```python
from build123d import *

# Parameters (mm, degrees)
ESQUISSE1_W                     = 20
ESQUISSE1_H                     = 20
BOSS_EXTRU_1_DEPTH              = 10
ESQUISSE2_W                     = 237.218260139
ESQUISSE2_H                     = 128.428413156
ENL_V_MAT_EXTRU_6_DEPTH         = 10
ENL_V_MAT_EXTRU_7_DEPTH         = 10
BOSS_EXTRU_4_START              = -2
BOSS_EXTRU_4_DEPTH              = 9
ESQUISSE10_W                    = 2
ESQUISSE10_H                    = 4
BOSS_EXTRU_5_DEPTH              = 224.980719072
ESQUISSE11_W                    = 2.5
ESQUISSE11_H                    = 5
BOSS_EXTRU_6_DEPTH              = 4
SYM_TRIE1_START                 = 8
SYM_TRIE1_OUTLINE_W             = 4
SYM_TRIE1_OUTLINE_H             = 4
SYM_TRIE1_DEPTH                 = 9
BOSS_EXTRU_9_REACH              = 128.238
BOSS_EXTRU_9_DIRECTION_2_REACH  = 128.238
BOSS_EXTRU_10_REACH             = 128.238
BOSS_EXTRU_10_DIRECTION_2_REACH = 128.238
ESQUISSE14_W                    = 8
ESQUISSE14_H                    = 8
BOSS_EXTRU_11_DEPTH             = 25


# Read off the part's stored shape, not the designer's step: Sym_trie1
with BuildPart() as part:
    # Esquisse1 → Boss.-Extru.1 (new body)
    with BuildSketch(Plane.XY):
        Polygon((-116.245179768, 65.5), (-116.245179768, 40.5), (-116.189357624, -40.5), (-116.189357624, -65.5), (108.67971716, -65.5), (108.67971716, -40.5), (108.735539304, 40.5), (108.735539304, 65.5), align=None)
        Polygon((83.754820232, 40.5), (106.172004788, 40.5), (106.172004788, -40.5), (83.67971716, -40.5), (83.67971716, -63), (-91.189357624, -63), (-91.189357624, -40.5), (-113.681645253, -40.5), (-113.681645253, 40.5), (-91.264460696, 40.5), (-91.264460696, 63), (83.754820232, 63), align=None, mode=Mode.SUBTRACT)
        Polygon((-113.66622051, -63.007706414), (-113.681645253, -43.007712371), (-93.681645253, -43.023131157), (-93.697069995, -62.992287629), align=None, mode=Mode.SUBTRACT)
        Polygon((106.172004788, -43.007712371), (106.156580046, -63.007706414), (86.187429531, -62.992287629), (86.172004788, -43.023131157), align=None, mode=Mode.SUBTRACT)
        with Locations((-103.754820232, 53)):
            Rectangle(ESQUISSE1_W, ESQUISSE1_H, mode=Mode.SUBTRACT)
        with Locations((96.245179768, 53)):
            Rectangle(ESQUISSE1_W, ESQUISSE1_H, mode=Mode.SUBTRACT)
    extrude(amount=BOSS_EXTRU_1_DEPTH)

    # Esquisse2 → Enl_v. mat.-Extru.6 (cut)
    with BuildSketch(Plane(origin=(0, 0, 0), x_dir=(-1, 0, 0), z_dir=(0, 0, -1))):
        with Locations((9.873590765, -23.714206578)):
            Rectangle(ESQUISSE2_W, ESQUISSE2_H)
    extrude(amount=-ENL_V_MAT_EXTRU_6_DEPTH, mode=Mode.SUBTRACT)

    # Esquisse4 → Enl_v. mat.-Extru.7 (cut)
    with BuildSketch(Plane(origin=(0, 0, 0), x_dir=(-1, 0, 0), z_dir=(0, 0, -1))):
        Polygon((-83.754820232, 63), (-83.754820232, 68.626436571), (91.264460696, 65.5), (91.264460696, 63), align=None)
    extrude(amount=-ENL_V_MAT_EXTRU_7_DEPTH, mode=Mode.SUBTRACT)


with BuildPart() as enl_v_mat_extru_7_piece_1:
    # of the separate pieces the step leaves, piece 1, a body of its own (enl_v_mat_extru_7_pieces)
    add(part.part.solids().sort_by_distance((-116.245179768, 65.5, 0))[0])

    # Esquisse9 → Boss.-Extru.4 (add)
    with BuildSketch(Plane.XY.offset(10).offset(BOSS_EXTRU_4_START)):
        Polygon((-116.245179768, 53), (-116.245179768, 55), (-120.245179768, 55), (-120.245179768, 51), (-116.245179768, 51), align=None)
    extrude(amount=BOSS_EXTRU_4_DEPTH)

    # Esquisse10 → Boss.-Extru.5 (add)
    with BuildSketch(Plane(origin=(-116.245179768, 0, 0), x_dir=(0, 0, -1), z_dir=(1, 0, 0))):
        with Locations((-16, 53)):
            Rectangle(ESQUISSE10_W, ESQUISSE10_H)
    extrude(amount=BOSS_EXTRU_5_DEPTH)

    # Esquisse11 → Boss.-Extru.6 (add)
    with BuildSketch(Plane.XZ.offset(-51)):
        with Locations((-114.995179768, 12.5)):
            Rectangle(ESQUISSE11_W, ESQUISSE11_H)
    extrude(amount=-BOSS_EXTRU_6_DEPTH)

    # Sym_trie1 outline → Sym_trie1 (add)
    with BuildSketch(Plane.XY.offset(SYM_TRIE1_START)):
        with Locations((-122.245179768, 53)):
            Rectangle(SYM_TRIE1_OUTLINE_W, SYM_TRIE1_OUTLINE_H)
    extrude(amount=SYM_TRIE1_DEPTH)


with BuildPart() as enl_v_mat_extru_7_piece_2:
    # of the separate pieces the step leaves, piece 2, a body of its own (enl_v_mat_extru_7_pieces)
    add(part.part.solids().sort_by_distance((108.735539304, 65.5, 0))[0])

    # Boss.-Extru.9: up to this face of the body (flat: up to its plane)
    boss_extru_9_end = Plane(enl_v_mat_extru_7_piece_2.part.faces().sort_by_distance((96.245179768, 65.5, 5))[0])
    # Esquisse12 → Boss.-Extru.9 (add, up to the picked face)
    with BuildSketch(Plane(origin=(0, 55, 0), x_dir=(1, 0, 0), z_dir=(0, 1, 0)), mode=Mode.PRIVATE) as boss_extru_9_sk1:
        Polygon((108.735539304, -10), (108.735539304, -8), (116.735539304, -8), (116.735539304, -17), (108.735539304, -17), (108.735539304, -15), (106.245539304, -15), (106.245539304, -10), align=None)
    boss_extru_9_tool1 = split(extrude(boss_extru_9_sk1.sketch, amount=BOSS_EXTRU_9_REACH, mode=Mode.PRIVATE), bisect_by=boss_extru_9_end, keep=Keep.BOTH, mode=Mode.PRIVATE)

    add(enl_v_mat_extru_7_piece_1.part)  # Boss.-Extru.9 merges Enl_v. mat.-Extru.7 piece 1
    add(boss_extru_9_tool1.solids().sort_by(Axis((111.962298, 55, 12.5), (0, 1, 0)))[0])

    # Boss.-Extru.9 direction 2: up to this face of the body (flat: up to its plane)
    boss_extru_9_direction_2_end = Plane(enl_v_mat_extru_7_piece_2.part.faces().sort_by_distance((96.245179768, 40.5, 5))[0])
    # Esquisse12 → Boss.-Extru.9 direction 2 (add, up to the picked face)
    with BuildSketch(Plane(origin=(0, 55, 0), x_dir=(1, 0, 0), z_dir=(0, 1, 0)), mode=Mode.PRIVATE) as boss_extru_9_direction_2_sk1:
        Polygon((108.735539304, -10), (108.735539304, -8), (116.735539304, -8), (116.735539304, -17), (108.735539304, -17), (108.735539304, -15), (106.245539304, -15), (106.245539304, -10), align=None)
    boss_extru_9_direction_2_tool1 = split(extrude(boss_extru_9_direction_2_sk1.sketch, amount=-BOSS_EXTRU_9_DIRECTION_2_REACH, mode=Mode.PRIVATE), bisect_by=boss_extru_9_direction_2_end, keep=Keep.BOTH, mode=Mode.PRIVATE)
    add(boss_extru_9_direction_2_tool1.solids().sort_by(Axis((111.962298, 55, 12.5), (0, -1, 0)))[0])

    # Boss.-Extru.10: up to this face of the body (flat: up to its plane)
    boss_extru_10_end = Plane(enl_v_mat_extru_7_piece_2.part.faces().sort_by_distance((100.216105898, 65.5, 6.894873222))[0])
    # Esquisse13 → Boss.-Extru.10 (add, up to the picked face)
    with BuildSketch(Plane(origin=(0, 55, 0), x_dir=(1, 0, 0), z_dir=(0, 1, 0)), mode=Mode.PRIVATE) as boss_extru_10_sk1:
        Polygon((-124.245179768, -17), (108.735539304, -17), (108.735539304, -15), (-113.745179768, -15), (-113.745179768, -10), (-116.245179768, -10), (-116.245179768, -8), (-124.245179768, -8), align=None)
    boss_extru_10_tool1 = split(extrude(boss_extru_10_sk1.sketch, amount=BOSS_EXTRU_10_REACH, mode=Mode.PRIVATE), bisect_by=boss_extru_10_end, keep=Keep.BOTH, mode=Mode.PRIVATE)
    add(boss_extru_10_tool1.solids().sort_by(Axis((-22.049518, 55, 15.446639), (0, 1, 0)))[0])

    # Boss.-Extru.10 direction 2: up to this face of the body (flat: up to its plane)
    boss_extru_10_direction_2_end = Plane(enl_v_mat_extru_7_piece_2.part.faces().sort_by_distance((-103.754820232, 40.5, 5))[0])
    # Esquisse13 → Boss.-Extru.10 direction 2 (add, up to the picked face)
    with BuildSketch(Plane(origin=(0, 55, 0), x_dir=(1, 0, 0), z_dir=(0, 1, 0)), mode=Mode.PRIVATE) as boss_extru_10_direction_2_sk1:
        Polygon((-124.245179768, -17), (108.735539304, -17), (108.735539304, -15), (-113.745179768, -15), (-113.745179768, -10), (-116.245179768, -10), (-116.245179768, -8), (-124.245179768, -8), align=None)
    boss_extru_10_direction_2_tool1 = split(extrude(boss_extru_10_direction_2_sk1.sketch, amount=-BOSS_EXTRU_10_DIRECTION_2_REACH, mode=Mode.PRIVATE), bisect_by=boss_extru_10_direction_2_end, keep=Keep.BOTH, mode=Mode.PRIVATE)
    add(boss_extru_10_direction_2_tool1.solids().sort_by(Axis((-22.049518, 55, 15.446639), (0, -1, 0)))[0])

    # Esquisse14 → Boss.-Extru.11 (add)
    with BuildSketch(Plane(origin=(0, 65.5, 0), x_dir=(1, 0, 0), z_dir=(0, 1, 0))):
        with Locations((112.735539304, -4)):
            Rectangle(ESQUISSE14_W, ESQUISSE14_H)
        with Locations((-120.245179768, -4)):
            Rectangle(ESQUISSE14_W, ESQUISSE14_H)
    extrude(amount=-BOSS_EXTRU_11_DEPTH)


solid = enl_v_mat_extru_7_piece_2.part
```
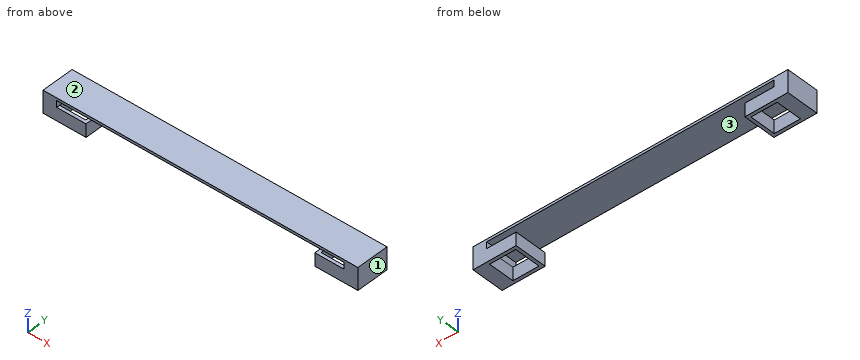
Geometry: final body of the model. Coordinates: model frame, mm. Face numbers are marked on the shaded views. Give positions to 0.01 mm unless a question says otherwise; leave off trailing zeros. Write each loop counter-clockwise with the first axis right and the second up, starting at its lowest first coordinate (ties: lowest second). Pieces come first, ordered by that corner, then holes.
1. Draft query along X for the marked faces 1, 2 and 3. Return one class per face: released by +X, released by -X, zero draft, split by the parting line, or undercut.
2. Section query B-B, the plane z = 12.5. Return loops of the section in (x, y).
3. Pin query (flat end, axial travel): P1, Ø6, axis at x = -85.5, z = 7, coming from the -Y side; P2, Ø12.5, axis at x = -58, y = 53, coming from the -Z side. Return the tip coordinate at first contact, or that it passes through.
4. Line query: probe 1 along X at (y, z) = (48.75, 5); probe 2 along X at (y, z) = (43.75, 12); probe 3 along Z at (x, y) = (-93, 45.25). Output: solid intervals per line, ascending.
5. Section query A-A, the plane x = -100. Return loops of the section in (y, z), then the cut area to 4 significant figures.
6. Section query C-C, the plane y = 49. Count the separate pieces of the cut face and the enclosed holes in it, then the cut area to 3 significant figures.
7. Section query D-D, the plane x = -14. Return loops of the section in (y, z).
Computed:
1. face 1: released by +X
1. face 2: zero draft
1. face 3: undercut
2. outline: (-124.25, 40.5) - (-113.75, 40.5) - (-113.75, 65.5) - (-124.25, 65.5) - close; (106.25, 40.5) - (116.74, 40.5) - (116.74, 65.5) - (106.25, 65.5) - close
3. P1: passes through
3. P2: stops at z = 15
4. probe 1: x = -124.25 to -113.75, -93.75 to -91.26, 83.75 to 86.25, 106.25 to 116.74
4. probe 2: x = -124.25 to -113.75, 106.25 to 116.74
4. probe 3: z = 0 to 10, 15 to 17
5. outline: (40.5, 0) - (43, 0) - (43, 10) - (40.5, 10) - close; (40.5, 15) - (65.5, 15) - (65.5, 17) - (40.5, 17) - close; (63, 0) - (65.5, 0) - (65.5, 10) - (63, 10) - close
5. area: 100.0 mm2
6. separate pieces: 3
6. enclosed holes: 0
6. area: 847 mm2
7. outline: (40.5, 15) - (65.5, 15) - (65.5, 17) - (40.5, 17) - close
